Verification items for the finished model (mm, model axes). A direction names the side the tool comes from. Give positions to 0.01 mm unless a question says otherwise; leave off trailing zeros. Loops run counter-clockwise (first coordinate to the right, second up) from the corner with the lowest first, then second, coordinate; pieces in that order, holes last. Notation, with made-up numbers: (60, 65) - (67, 65) arc R20 ccw to (67, 83) - close; hole circle Ø10 at (2, 9.5). An arc over 180 degrees is marked (long way). Answer in a Markdown table with one row per item.
```python
from build123d import *

# Parameters (mm, degrees)
F1_DEPTH = 41.275
F2_R     = 9.525
F3_DEPTH = 53.34
F5_DEPTH = 55.372
F6_R     = 2.271843
F7_DEPTH = 106.934
F8_R     = 2.155263
F9_DEPTH = 91.948


with BuildPart() as f1:
    # F0 (on Front) → F1 (new body)
    with BuildSketch(Plane.XZ):
        Polygon((237.607324, -13.441301), (-67.192676, 29.738699), (-67.192676, -33.761301), (237.607324, -33.761301), align=None)
    extrude(amount=-F1_DEPTH)

    # F2 (on face) → F3 (cut)
    with BuildSketch(Plane(origin=(-67.192676, 0, 0), x_dir=(0, -1, 0), z_dir=(-1, 0, 0))):
        with Locations((-20.6375, -2.011301)):
            Circle(F2_R)
    extrude(amount=-F3_DEPTH, mode=Mode.SUBTRACT)

    # F4 (on face) → F5 (cut)
    with BuildSketch(Plane.XZ):
        Polygon((237.607324, -13.441301), (-67.192676, 29.738699), (75.7569, 0), align=None)
    extrude(amount=-F5_DEPTH, mode=Mode.SUBTRACT)

    # F6 (on Front) → F7 (cut)
    with BuildSketch(Plane.XZ):
        with Locations((9.710665, -28.575001)):
            Circle(F6_R)
    extrude(amount=-F7_DEPTH, mode=Mode.SUBTRACT)

    # F8 (on face) → F9 (cut)
    with BuildSketch(Plane.XZ):
        with Locations((181.414664, -29.591002)):
            Circle(F8_R)
    extrude(amount=-F9_DEPTH, mode=Mode.SUBTRACT)


solid = f1.part
```
Q1. Sectioned sample at B-B (y = 17). Record the cut outline in (x, z) (1 decimal).
Completed:
| item | result |
|---|---|
| outline | (-67.2, -33.8) - (237.6, -33.8) - (237.6, -13.4) - (75.8, 0) - (-67.2, 29.7) - (-67.2, 6.8) - (-13.9, 6.8) - (-13.9, -10.8) - (-67.2, -10.8) - close; hole circle Ø4.5 at (9.7, -28.6); hole circle Ø4.3 at (181.4, -29.6) |
Q2. Sectioned sample at A-A (y = 3.5). Record the cut outline in (x, z) (1 decimal), and give its area (3 significant figures).
Completed:
| item | result |
|---|---|
| outline | (-67.2, -33.8) - (237.6, -33.8) - (237.6, -13.4) - (75.8, 0) - (-67.2, 29.7) - close; hole circle Ø4.5 at (9.7, -28.6); hole circle Ø4.3 at (181.4, -29.6) |
| area | 11,300 mm^2 |
Q3. Sectioned sample at D-D (x = 24.5). Record the cut outline in (y, z) (3 decimals), and give its area (3 significant figures).
Completed:
| item | result |
|---|---|
| outline | (0, -33.761) - (41.275, -33.761) - (41.275, 10.663) - (0, 10.663) - close |
| area | 1,830 mm^2 |
Q4. Thickness scan on line 1 (Z direction, x = -24.5, y = 25); line 2 (Y direction, x = -26, z = 4.5) (3 decimals); line 3 (Z direction, x = 211.5, y = 20.5). Record the ranges inside material, lowest first.
Completed:
| item | result |
|---|---|
| line 1 | -33.76 to -10.48, 6.46 to 20.86 |
| line 2 | 0 to 13.686, 27.589 to 41.275 |
| line 3 | -33.76 to -11.27 |
Q5. Sectioned sample at C-C (z = -6.5). Record the cut outline in (x, y) (3 decimals), and give its area (3 significant figures).
Completed:
| item | result |
|---|---|
| outline | (-67.193, 0) - (154.025, 0) - (154.025, 41.275) - (-67.193, 41.275) - (-67.193, 29.039) - (-13.853, 29.039) - (-13.853, 12.236) - (-67.193, 12.236) - close |
| area | 8,230 mm^2 |
Q6. Draft check along Z on faces 1 (the face through (-13.853, 21, -2)), 2 (the face through (49, 41.275, -9)), 3 (the face through (155.549, 20.349, -6.627)). Enter one of: +Z half, -Z half, draft (parallel to the pull), parting line (faces both ways), or undercut.
Completed:
| item | result |
|---|---|
| face 1 | undercut |
| face 2 | draft |
| face 3 | +Z half |
Q7. Go/stop test with a flat-tipped pin: P1, Ø9.5, axis at y = 20, z = -6, coming from the -X side. Record where the tip stops, or that it passes through.
Completed:
| item | result |
|---|---|
| P1 | x = -13.85 |
Q8. Tool access check on faces 4 (the face through (-40.896, 11.552, 0.85)), 5 (the face through (237.607, 20, -24)). Record the directions out of +Z, -Z, +X, -X, +Y, -Y that give a thin tool (end or side, any length) a straight path to the whole face; none if there is none.
Completed:
| item | result |
|---|---|
| face 4 | -X |
| face 5 | +Z, -Z, +X, +Y, -Y |
